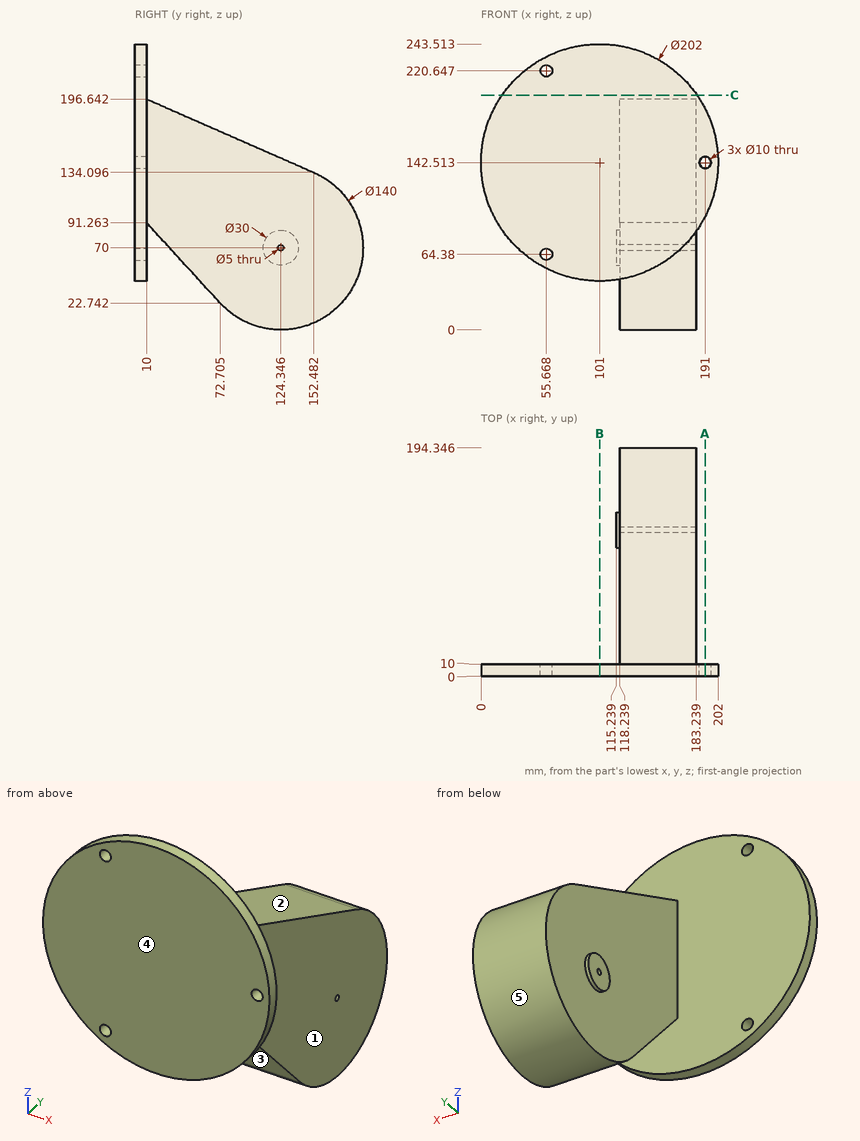
Verification items for this drawing (mm, ordinates from the low corner). A direction names the side the tool comes from. Round coordinates to 2 decimals unless told otherwise and drop trailing zeros. Order: outer loops, then holes, each group sorted by start corner. A loop starts at its lowest first (then second) coordinate and runs counter-clockwise, first axis right, second up. Notation, with made-up numbers: (58, 68) - (65, 68) arc R36 cw to (65, 105) - close; hole circle Ø10 at (-40, 88.25). An arc over 180 degrees is marked (long way). Answer as CSV lines item,"result". Start each with the question number.
1) Scan lines: probe 1 along X at (y, z) = (63, 43.5); probe 2 along Y at (x, z) = (110, 62.5); probe 3 along Y at (x, z) = (154.5, 78.5). Record each from-to range of solid material in increasing order.
2) Section check A-A (x = 191). Record the cut outline in (y, z), then the cut area to 3 significant figures.
3) Section check C-C (z = 200). Record the cut outline in (x, y).
4) Tool access check on the marked faces 1 and 2. Record the directions out of +Z, -Z, +X, -X, +Y, -Y that give a thin tool (end or side, any length) a straight path to the whole face; none if there is none.
5) Draft check along Y on the marked faces 3, 4 and 5. Enter one of: +Y half, -Y half, draft (parallel to the pull), parting line (faces both ways), or undercut.
6) Section check B-B (x = 101). Record the cut outline in (y, z), then the cut area to 3 significant figures.
7) Depth check by flat-ended pin: pin 1 (3 mm diameter, centred on x = 32, z = 126, fed in from -Y); pin 2 (10 mm diameter, centred on x = 120, y = 104, fed in from -Z); pin 3 (6 mm diameter, centred on y = 120.5, z = 127.5, fed in from -X); pin 4 (24 mm diameter, centred on y = 121, z = 74.5, fed in from -X). Enter the tip coordinate at first touch or a pass-through.
Determined:
1,probe 1,"118.24 to 183.24"
1,probe 2,"0 to 10"
1,probe 3,"0 to 10, 21.68 to 193.83"
2,outline,"(0, 96.68) - (10, 96.68) - (10, 137.51) - (0, 137.51) - close; (0, 147.51) - (10, 147.51) - (10, 188.35) - (0, 188.35) - close"
2,area,"817 mm^2"
3,outline,"(17.96, 0) - (184.04, 0) - (184.04, 10) - (17.96, 10) - close"
4,face 1,"+Z, -Z, +X, +Y"
4,face 2,"+Z, +X, -X, +Y"
5,face 3,"undercut"
5,face 4,"-Y half"
5,face 5,"parting line"
6,outline,"(0, 41.51) - (10, 41.51) - (10, 243.51) - (0, 243.51) - close"
6,area,"2,020 mm^2"
7,pin 1,"y = 0"
7,pin 2,"z = 1.7"
7,pin 3,"x = 118.24"
7,pin 4,"x = 115.24"
